Job drawing, mm, ordinate dimensions from the low corner. One solid piece. Give positions to 0.01 mm unless a question says otherwise; leave off trailing zeros. Order: outer loops, then holes, each group sorted by start corner. A loop starts at its lowest first (then second) coordinate and runs counter-clockwise, first axis right, second up.
1. Slice it at B-B on z = 54. List the corners of the cut face in (x, y) (1 decimal).
2. Slice it at D-D on z = 82. List the corners of the cut face in (x, y) (1 decimal), and give its area (3 significant figures).
3. Slice it at C-C on y = 4.25. Give the number of separate pieces and of enclosed holes in the cut face, and give its area (3 significant figures).
4. Probe line 1 (X direction, y = 7.75, z = 57.5); line 2 (X direction, y = 6, z = 7) (1 decimal); line 3 (X direction, y = 6, z = 51) (1 decimal). List the from-to ranges inside material, lowest first.
5. Slice it at A-A on z = 15. List the corners of the cut face in (x, y) (1 decimal).
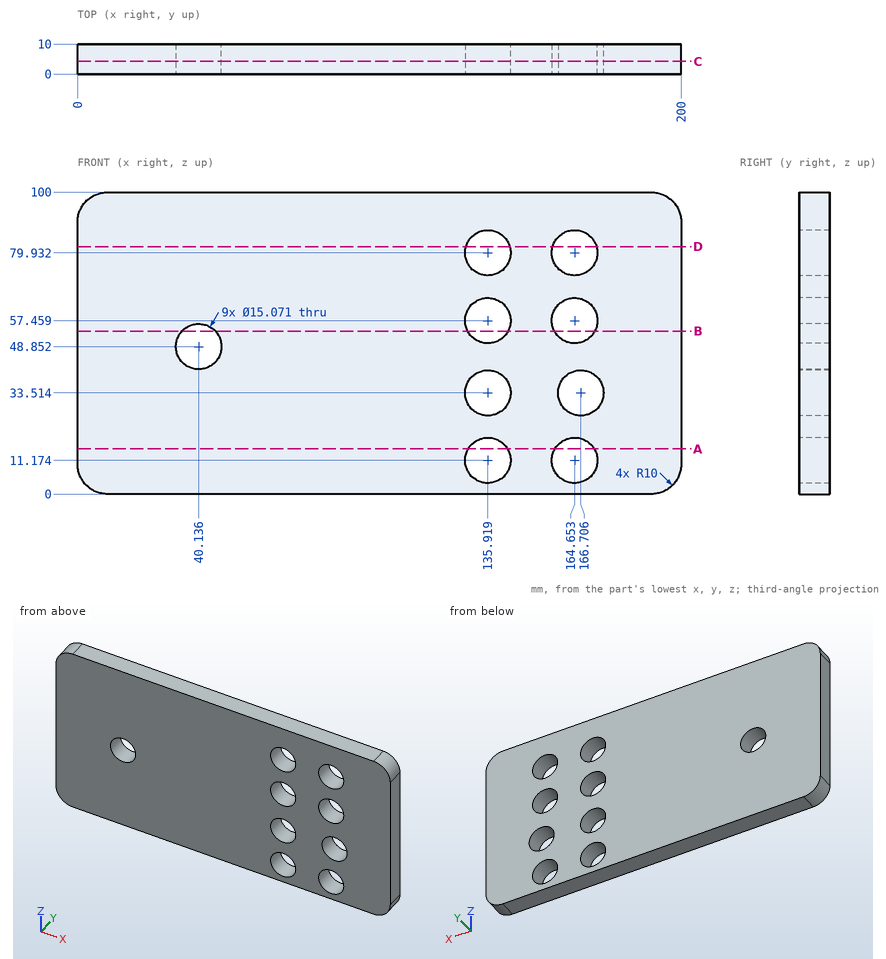
Data:
1. outline: (0, 0) - (34.6, 0) - (34.6, 10) - (0, 10) - close; (45.6, 0) - (129.2, 0) - (129.2, 10) - (45.6, 10) - close; (142.6, 0) - (158, 0) - (158, 10) - (142.6, 10) - close; (171.3, 0) - (200, 0) - (200, 10) - (171.3, 10) - close
2. outline: (0, 0) - (128.7, 0) - (128.7, 10) - (0, 10) - close; (143.2, 0) - (157.4, 0) - (157.4, 10) - (143.2, 10) - close; (171.9, 0) - (200, 0) - (200, 10) - (171.9, 10) - close
2. area: 1,710 mm2
3. separate pieces: 1
3. enclosed holes: 9
3. area: 18,300 mm2
4. line 1: x = 0 to 128.38, 143.45 to 157.12, 172.19 to 200
4. line 2: x = 0.5 to 129.6, 142.2 to 158.4, 170.9 to 199.5
4. line 3: x = 0 to 32.9, 47.4 to 132, 139.8 to 160.8, 168.5 to 200
5. outline: (0, 0) - (129.4, 0) - (129.4, 10) - (0, 10) - close; (142.4, 0) - (158.2, 0) - (158.2, 10) - (142.4, 10) - close; (171.1, 0) - (200, 0) - (200, 10) - (171.1, 10) - close
